```python
from build123d import *

# Parameters (mm, degrees)
BOSS_EXTRUDE8_DEPTH                                  = 1.5
BOSS_EXTRUDE9_START                                  = -1.5
BOSS_EXTRUDE9_DEPTH                                  = 1.5
BOSS_EXTRUDE10_DEPTH                                 = 1
CHAMFER2_SIZE                                        = 1
CUT_EXTRUDE6_DEPTH                                   = 28.162128967
CHAMFER5_SIZE                                        = 1.249835708
CHAMFER5_SIZE_2                                      = 1
CSK_FOR_M1_6_COUNTERSUNK_FLAT_HEAD_SCREW_D           = 1.8
CSK_FOR_M1_6_COUNTERSUNK_FLAT_HEAD_SCREW_DEPTH       = 2.5
CSK_FOR_M1_6_COUNTERSUNK_FLAT_HEAD_SCREW_CSINK_D     = 3.6
CSK_FOR_M1_6_COUNTERSUNK_FLAT_HEAD_SCREW_CSINK_ANGLE = 90
CSK_FOR_M1_6_COUNTERSUNK_FLAT_HEAD_SCREW_TIP         = 0.540774557


with BuildPart() as part:
    # Sketch15 → Boss-Extrude8 (new body)
    with BuildSketch(Plane(origin=(0, 0, 0), x_dir=(1, 0, 0), z_dir=(0, 1, 0))):
        with BuildLine():
            Line((0, 0), (-15.625, 0))
            ThreePointArc((-15.625, 0), (-7.8125, 13.531646934), (7.8125, 13.531646934))
            Line((7.8125, 13.531646934), (0, 0))
        make_face()
    extrude(amount=BOSS_EXTRUDE8_DEPTH)



with BuildPart() as body_2:
    # Sketch16 → Boss-Extrude9 (new body)
    with BuildSketch(Plane(origin=(0, 1.5, 0), x_dir=(1, 0, 0), z_dir=(0, 1, 0)).offset(BOSS_EXTRUDE9_START)):
        with BuildLine():
            Line((2.020725942, -3.5), (12.432094511, 14.533019338))
            ThreePointArc((12.432094511, 14.533019338), (-9.5625, 16.562735847), (-18.802011196, -3.5))
            Line((-18.802011196, -3.5), (2.020725942, -3.5))
        make_face()
        with BuildLine():
            Line((0.866025404, -1.5), (9.828628146, 14.023683317))
            ThreePointArc((9.828628146, 14.023683317), (-8.5625, 14.83068504), (-17.05918008, -1.5))
            Line((-17.05918008, -1.5), (0.866025404, -1.5))
        make_face(mode=Mode.SUBTRACT)
    extrude(amount=BOSS_EXTRUDE9_DEPTH)


with BuildPart() as part_1:
    add(part.part)

    add(body_2.part)  # Boss-Extrude10 merges body 2
    # Sketch17 → Boss-Extrude10 (add)
    with BuildSketch(Plane.XZ):
        with BuildLine():
            Line((12.432094511, -14.533019338), (2.020725942, 3.5))
            Line((2.020725942, 3.5), (-18.802011196, 3.5))
            ThreePointArc((-18.802011196, 3.5), (-9.5625, -16.562735847), (12.432094511, -14.533019338))
        make_face()
    extrude(amount=BOSS_EXTRUDE10_DEPTH)

    # Chamfer2
    # the kernel refuses this chamfer: 1 mm, written as the material it takes off along each edge
    with BuildSketch(Plane(origin=(-15.625, 0, 0), x_dir=(1, 0, 0), z_dir=(0, 1, 0))) as chamfer2_piece_1:
        with BuildLine():
            Line((CHAMFER2_SIZE, 0), (0.030129793, 0.969870207))
            ThreePointArc((0.030129793, 0.969870207), (0.007965345, 0.498852279), (0, 0))
            Line((0, 0), (CHAMFER2_SIZE, 0))
        make_face()
    extrude(amount=4.071682988, mode=Mode.SUBTRACT)
    with BuildSketch(Plane(origin=(7.8125, 0, -13.531646934), x_dir=(-0.8811332220086912, 0, -0.4728681053661608), z_dir=(0, 1, 0))) as chamfer2_piece_2:
        with BuildLine():
            Line((0.970338097, 0), (CHAMFER2_SIZE * 0.0310508191178, CHAMFER2_SIZE * 0.999517807061))
            Line((CHAMFER2_SIZE * 0.0310508191178, CHAMFER2_SIZE * 0.999517807061), (0, 0))
            ThreePointArc((0, 0), (0.498859067, -0.007528267), (0.970338097, 0))
        make_face()
    extrude(amount=4.071682988, mode=Mode.SUBTRACT)

    # Sketch19 → Cut-Extrude6 (cut, through all)
    with BuildSketch(Plane(origin=(0, 1.5, 0), x_dir=(1, 0, 0), z_dir=(0, 1, 0))):
        Polygon((-0.133974596, -1.5), (-0.133974596, -3.5), (2.020725942, -3.5), (3.098076211, -1.633974596), (1.366025404, -0.633974596), (0.866025404, -1.5), align=None)
    extrude(amount=-CUT_EXTRUDE6_DEPTH, mode=Mode.SUBTRACT)

    # Chamfer5
    # the kernel refuses this chamfer: 1.249835708, 1 mm, written as the material it takes off along each edge
    with BuildSketch(Plane(origin=(12.432094511, -4.228421452, -14.533019338), x_dir=(-0.500000000000006, 0, 0.8660254037844353), z_dir=(0, 1, 0))) as chamfer5_piece_1:
        with BuildLine():
            Line((CHAMFER5_SIZE, 0), (-0.153998799, -0.963208706))
            ThreePointArc((-0.153998799, -0.963208706), (-0.08585038, -0.497615929), (0, 0))
            Line((0, 0), (CHAMFER5_SIZE, 0))
        make_face()
    extrude(amount=8.956842905, mode=Mode.SUBTRACT)
    with BuildSketch(Plane(origin=(-18.802011196, -4.09148885, 3.5), x_dir=(-0.1521791167983569, 0, -0.9883529310982349), z_dir=(0, 1, 0))) as chamfer5_piece_2:
        with BuildLine():
            Line((1.195923602, 0), (-CHAMFER5_SIZE_2 * 0.152179116798, -CHAMFER5_SIZE_2 * 0.988352931098))
            Line((-CHAMFER5_SIZE_2 * 0.152179116798, -CHAMFER5_SIZE_2 * 0.988352931098), (0, 0))
            ThreePointArc((0, 0), (0.618115367, 0.009339597), (1.195923602, 0))
        make_face()
    extrude(amount=8.6829777, mode=Mode.SUBTRACT)

    # CSK for M1.6 Countersunk Flat Head Screw1
    with Locations(Plane(origin=(0, 1.5, 0), x_dir=(1, 0, 0), z_dir=(0, 1, 0))):
        with Locations((-3.65625, 6.332810765), (-9.718427826, 2.832810765), (2.405927826, 9.832810765)):
            CounterSinkHole(CSK_FOR_M1_6_COUNTERSUNK_FLAT_HEAD_SCREW_D / 2, CSK_FOR_M1_6_COUNTERSUNK_FLAT_HEAD_SCREW_CSINK_D / 2, depth=CSK_FOR_M1_6_COUNTERSUNK_FLAT_HEAD_SCREW_DEPTH, counter_sink_angle=CSK_FOR_M1_6_COUNTERSUNK_FLAT_HEAD_SCREW_CSINK_ANGLE)
            with Locations((0, 0, -(CSK_FOR_M1_6_COUNTERSUNK_FLAT_HEAD_SCREW_DEPTH + CSK_FOR_M1_6_COUNTERSUNK_FLAT_HEAD_SCREW_TIP / 2))):  # 118° drill point
                Cone(0, CSK_FOR_M1_6_COUNTERSUNK_FLAT_HEAD_SCREW_D / 2, CSK_FOR_M1_6_COUNTERSUNK_FLAT_HEAD_SCREW_TIP, mode=Mode.SUBTRACT)


solid = part_1.part
```
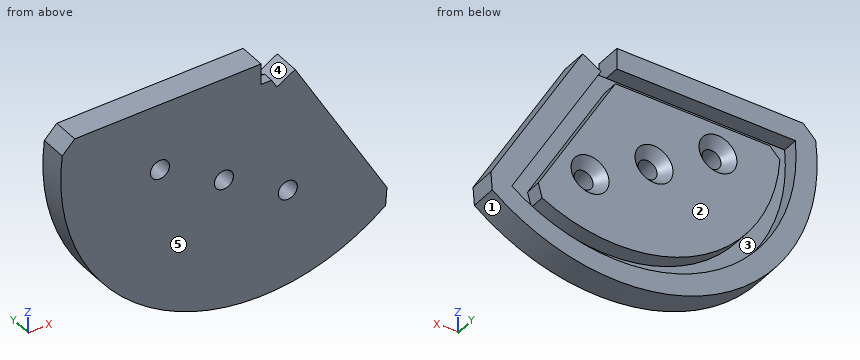
Geometry check sheet. Reference: the model listing, model coordinates, mm. Face numbers are marked on the shaded views. A direction names the side the tool comes from. Give positions to 0.01 mm unless a question says otherwise; leave off trailing zeros. Write each loop counter-clockwise with the first axis right and the second up, starting at its lowest first coordinate (ties: lowest second). Pieces come first, ordered by that corner, then holes. Notation, with made-up numbers: (34.25, 68) -> (84.25, 68) arc R23 cw to (84.25, 88) -> close; hole circle Ø7 at (4, -24.5). An arc over 180 degrees is marked (long way). One line per question, with ' | ' between items.
Item 1: Sectioned sample at C-C, the plane x = -16.5. Record the boundary of the cut face in (y, z), plus the area to 3 significant figures.
Determined:
outline: (-1, -9.67) -> (1.5, -9.67) -> (1.5, -4.58) -> (0, -4.58) -> (0, 1.5) -> (1.5, 1.5) -> (1.5, 3.5) -> (-1, 3.5) -> close | area: 23.8 mm^2
Item 2: Sectioned sample at D-D, the plane z = -16.5. Record the boundary of the cut face in (x, y), plus the area to 3 significant figures.
Determined:
outline: (-9.67, -1) -> (9.67, -1) -> (9.67, 1.5) -> (4.58, 1.5) -> (4.58, 0) -> (-4.58, 0) -> (-4.58, 1.5) -> (-9.67, 1.5) -> close | area: 34.6 mm^2
Item 3: Access from +Z, -Z, +X, -X, +Y, -Y to the whole of each face (thin tool, end or side, straight path). Record for the marked faces 4 and 5.
Determined:
face 4: +Z, +Y, -Y | face 5: +Z, -Z, +X, -X, -Y
Item 4: Draft check along X on the marked faces 1, 2 and 3. Enter one of: released by +X, released by -X, zero draft, split by the parting line, or undercut.
Determined:
face 1: split by the parting line | face 2: zero draft | face 3: undercut
Item 5: Scan lines: line 1 along Z through (x, y) = (4, 0.1); line 2 along X through (y, z) = (1.3, -12.75); line 3 along Z through (x, y) = (-7.5, 0.3). Record each from-to range of solid material in increasing order.
Determined:
line 1: -18.7 to -16.65, -15.1 to -6.93, -3.93 to 0.07 | line 2: -14.25 to -11.43, -9.03 to 7.29, 9.09 to 11.4 | line 3: -17.59 to -15.4, -13.71 to 0, 1.5 to 3.5
Item 6: Sectioned sample at A-A, the plane y = -0.4. Record the boundary of the cut face in (x, z) (3 decimals), plus the area to 3 significant figures.
Determined:
outline: (-18.984, 2.318) arc R19.125 ccw to (11.675, -15.148) -> (11.807, -13.451) -> (3.098, 1.634) -> (1.366, 0.634) -> (0.866, 1.5) -> (-0.134, 1.5) -> (-0.134, 3.5) -> (-17.802, 3.5) -> close; hole circle Ø1.8 at (-9.718, -2.833); hole circle Ø1.8 at (-3.656, -6.333); hole circle Ø1.8 at (2.406, -9.833) | area: 508 mm^2
Item 7: Sectioned sample at B-B, the plane z = 1. Record the boundary of the cut face in (x, y), plus the area to 3 significant figures.
Determined:
outline: (-19.1, -1) -> (1.15, -1) -> (1.15, 0) -> (-17.1, 0) -> (-17.1, 1.5) -> (-19.1, 1.5) -> close; (2, -1) -> (3.46, -1) -> (3.46, 1.5) -> (2, 1.5) -> close | area: 26.9 mm^2
Item 8: Depth check by flat-ended pin: pin 1 (0.8 mm diameter, centred on x = 0.5, y = -0.5, fed in from +Z); pin 2 (2 mm diameter, centred on x = -3.66, z = -6.33, fed in from +Y). Enter the tip coordinate at first touch or a pass-through.
Determined:
pin 1: z = 1.5 | pin 2: y = 0.7
